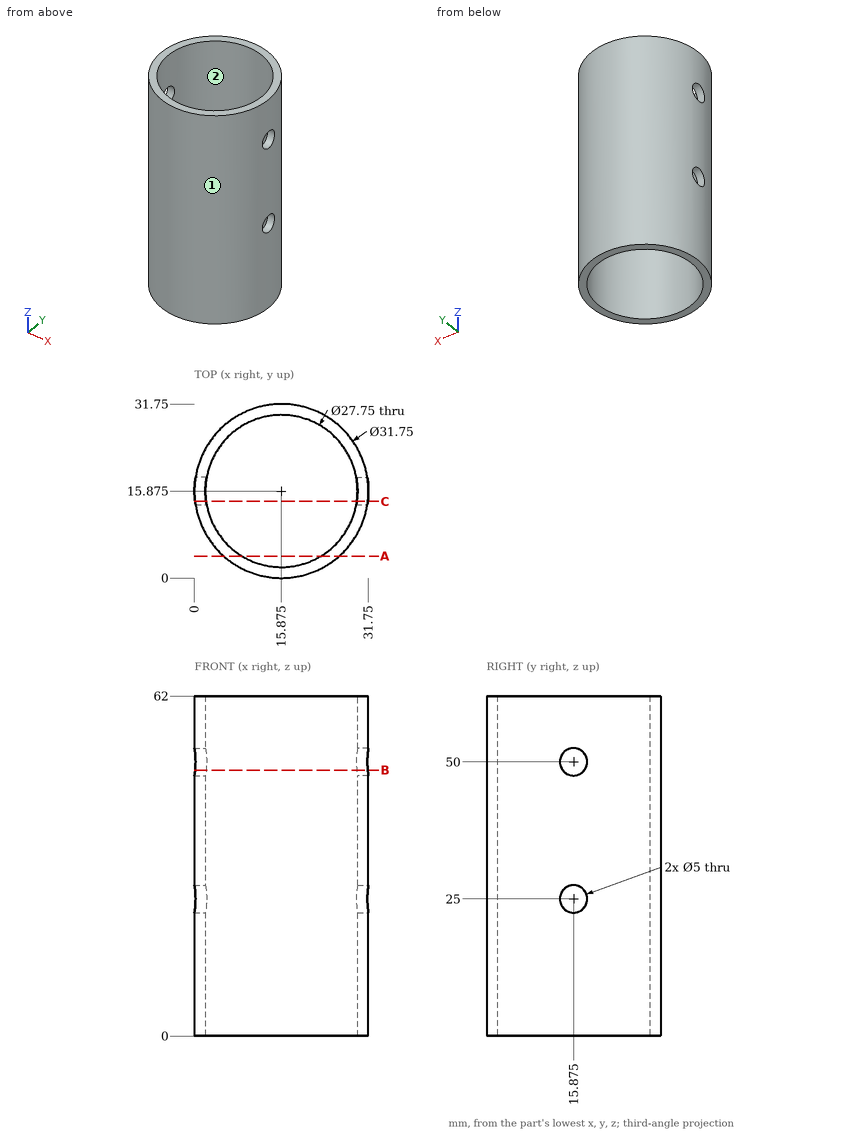
Drawing for the job (mm, zero at the part's lowest x, y, z). Coordinates: 2 decimals unless noted, no trailing zeros. Loops run counter-clockwise (first coordinate to the right, second up) from the corner with the lowest first, then second, coordinate; pieces in that order, holes last. Notation, with made-up numbers: (39, -10.75) - (52, -10.75) arc R34 ccw to (52, 22.25) - close; hole circle Ø11 at (20.5, -6.5). An arc over 180 degrees is marked (long way). Return JSON: item names as keys, results as strings.
1. Mould opens along X. For the marked faces 1 and 2 say: released by +X, released by -X, zero draft, split by the parting line, or undercut.
Result:
{"face 1": "split by the parting line", "face 2": "undercut"}
2. Band-saw the part on C-C (y = 14). Give the cut face in (x, z).
Result:
{"outline": "(0.11, 0) - (2.13, 0) - (2.13, 23.35) - (0.11, 23.35) - close; (0.11, 26.65) - (2.13, 26.65) - (2.13, 48.35) - (0.11, 48.35) - close; (0.11, 51.65) - (2.13, 51.65) - (2.13, 62) - (0.11, 62) - close; (29.62, 0) - (31.64, 0) - (31.64, 23.35) - (29.62, 23.35) - close; (29.62, 26.65) - (31.64, 26.65) - (31.64, 48.35) - (29.62, 48.35) - close; (29.62, 51.65) - (31.64, 51.65) - (31.64, 62) - (29.62, 62) - close"}
3. Band-saw the part on A-A (y = 4). Give the cut face in (x, z), and give its area (3 significant figures).
Result:
{"outline": "(5.34, 0) - (8.7, 0) - (8.7, 62) - (5.34, 62) - close; (23.05, 0) - (26.41, 0) - (26.41, 62) - (23.05, 62) - close", "area": "417 mm2"}
4. Drop flat-ended pins along their axis: pin 1 (10 mm diameter, centred on y = 6.5, z = 44, fed in from +X); pin 2 (12 mm diameter, centred on x = 6.5, z = 33.5, fed in from +Y); pin 3 (4 mm diameter, centred on y = 15.875, z = 50, fed in from +X); pin 4 (8 mm diameter, centred on y = 25, z = 52.5, fed in from -X). Give the stop position or say it passes through.
Result:
{"pin 1": "stops at x = 31.14", "pin 2": "stops at y = 31.39", "pin 3": "passes through", "pin 4": "stops at x = 0.85"}
5. Band-saw the part on B-B (z = 48.5). Give the cut face in (x, y) (3 decimals), and give its area (3 significant figures).
Result:
{"outline": "(0.126, 13.875) arc R15.875 ccw to (31.624, 13.875) - (29.605, 13.875) arc R13.875 cw to (2.145, 13.875) - close; (0.126, 17.875) - (2.145, 17.875) arc R13.875 cw to (29.605, 17.875) - (31.624, 17.875) arc R15.875 ccw to start", "area": "171 mm2"}
6. Probe L1, parallel to Y at x = 15.5, z = 56; L2, parallel to X at y = 19, z = 10; L3, parallel to X at y = 5.5, z = 52.5. List the from-to ranges inside material, lowest first. Write a range as from..to.
Result:
{"L1": "y = 0..2.01, 29.74..31.75", "L2": "x = 0.31..2.36, 29.39..31.44", "L3": "x = 3.86..6.66, 25.09..27.89"}
